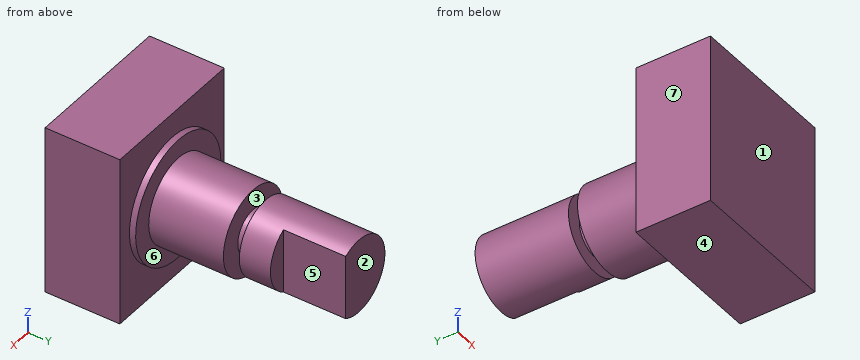
from build123d import *

# Parameters (mm, degrees)
SKETCH2_W           = 3
SKETCH2_H           = 5.196152422
CUT_EXTRUDE1_DEPTH  = 5
SKETCH3_W           = 12
SKETCH3_H           = 13.7
BOSS_EXTRUDE1_DEPTH = 6


with BuildPart() as part:
    # Sketch1 → Revolve1 (revolve)
    with BuildSketch(Plane.XY, mode=Mode.PRIVATE) as revolve1_sk:
        Polygon((0, 15), (-3, 15), (-3, 7.5), (-1.75, 7.5), (-1.75, 6.5), (-3.4, 6.5), (-3.4, 0.5), (-4.9, 0.5), (-4.9, 0), (0, 0), align=None)
    revolve(revolve1_sk.sketch.rotate(Axis((0, 0, 0), (0, 1, 0)), 270), axis=Axis((0, 0, 0), (0, 1, 0)))

    # Sketch2 → Cut-Extrude1 (cut)
    with BuildSketch(Plane(origin=(0, 15, 0), x_dir=(1, 0, 0), z_dir=(0, 1, 0))):
        with Locations((3, 0)):
            Rectangle(SKETCH2_W, SKETCH2_H)
    extrude(amount=-CUT_EXTRUDE1_DEPTH, mode=Mode.SUBTRACT)

    # Sketch3 → Boss-Extrude1 (add)
    with BuildSketch(Plane(origin=(0, 0, 0), x_dir=(-1, 0, 0), z_dir=(0, -1, 0))):
        Rectangle(SKETCH3_W, SKETCH3_H)
    extrude(amount=BOSS_EXTRUDE1_DEPTH)


solid = part.part
Source: CAD feature listing. Evaluate the final solid. Frame: model axes, mm. Face numbers are marked on the shaded views. A direction names the side the tool comes from. Round coordinates to 2 decimals unless told otherwise and drop trailing zeros. Loops run counter-clockwise (first coordinate to the right, second up) from the corner with the lowest first, then second, coordinate; pieces in that order, holes last.
Q1. Ray query, line 1 (Y direction, x = -5, z = 0); line 2 (Y direction, x = 3.75, z = 0); line 3 (X direction, y = 11.75, z = 1.5). Return the intervals inside material, ascending.
Q2. Mould query, pull axis Y, two halves, no side actions, for the marked faces 1, 2, 3 and 4. Classes: pulls with the +Y half, pulls with the -Y half, needs draft (parallel to the pull), parting line crosses it, or undercut.
Q3. Section B-B, the plane z = -2.25. Return loops of the section in (x, y), plus the area to 3 significant figures.
Q4. Access query for the marked faces 5, 6 and 7. Directions: +Z, -Z, +X, -X, +Y, -Y. A direction counts if a zero-diameter tool reaches every point of the face in a straight line with its end or side. Return the directions, or none.
Q5. Section C-C, the plane z = 0. Return loops of the section in (x, y).
Q6. Section D-D, the plane y = 12.75. Return loops of the section in (x, z), plus the area to 3 significant figures.
Q7. Section A-A, the plane x = 0. Return loops of the section in (y, z).
Q8. First-contact query: P1, Ø2.5, axis at y = 12, z = 0, coming from the +X side; P2, Ø4, axis at y = 8, z = -3, coming from the +X side; P3, Ø1, axis at y = 3, z = -1.5, coming from the +X side. Flat tips, straight axial feed; report the tip coordinate or a pass-through.
Solutions:
1. line 1: y = -6 to 0
1. line 2: y = -6 to 0.5
1. line 3: x = -2.6 to 1.5
2. face 1: pulls with the -Y half
2. face 2: pulls with the +Y half
2. face 3: undercut
2. face 4: needs draft
3. outline: (-6, -6) - (6, -6) - (6, 0) - (4.35, 0) - (4.35, 0.5) - (2.55, 0.5) - (2.55, 6.5) - (-2.55, 6.5) - (-2.55, 0.5) - (-4.35, 0.5) - (-4.35, 0) - (-6, 0) - close; (-1.98, 7.5) - (1.98, 7.5) - (1.98, 10) - (1.5, 10) - (1.5, 15) - (-1.98, 15) - close
3. area: 134 mm2
4. face 5: +Z, -Z, +X, +Y
4. face 6: +Y
4. face 7: +Z, -Z, -X, +Y, -Y
5. outline: (-6, -6) - (6, -6) - (6, 0) - (4.9, 0) - (4.9, 0.5) - (3.4, 0.5) - (3.4, 6.5) - (1.75, 6.5) - (1.75, 7.5) - (3, 7.5) - (3, 10) - (1.5, 10) - (1.5, 15) - (-3, 15) - (-3, 7.5) - (-1.75, 7.5) - (-1.75, 6.5) - (-3.4, 6.5) - (-3.4, 0.5) - (-4.9, 0.5) - (-4.9, 0) - (-6, 0) - close
6. outline: (1.5, -2.6) - (1.5, 2.6) arc R3 ccw (long way) to start
6. area: 22.7 mm2
7. outline: (-6, -6.85) - (0, -6.85) - (0, -4.9) - (0.5, -4.9) - (0.5, -3.4) - (6.5, -3.4) - (6.5, -1.75) - (7.5, -1.75) - (7.5, -3) - (15, -3) - (15, 3) - (7.5, 3) - (7.5, 1.75) - (6.5, 1.75) - (6.5, 3.4) - (0.5, 3.4) - (0.5, 4.9) - (0, 4.9) - (0, 6.85) - (-6, 6.85) - close
8. P1: stops at x = 1.5
8. P2: stops at x = 2.96
8. P3: stops at x = 3.25
